Build history of the part. All positions in model axes, mm. Round coordinates to 2 decimals unless told otherwise and drop trailing zeros. Loops run counter-clockwise (first coordinate to the right, second up) from the corner with the lowest first, then second, coordinate; pieces in that order, holes last. Notation, with made-up numbers: (61, 18.5) - (82, 18.5) arc R17 ccw to (82, 47.5) - close; hole circle Ø3 at (29, 24.5). An arc over 180 degrees is marked (long way). One line per question, with ' | ' between items. Start each with the question number.
from build123d import *

# Parameters (mm, degrees)
SKETCH_1_R          = 15
EXTRUDE_1_DEPTH     = 3
M3X0_5_1_D          = 2.5
SKETCH_6_R          = 3
CUT_EXTRUDE_2_DEPTH = 22.424285286


with BuildPart() as part:
    # ｽｹｯﾁ1 → ﾎﾞｽ - 押し出し1 (new body)
    with BuildSketch(Plane(origin=(0, 0, 0), x_dir=(0, 0, -1), z_dir=(1, 0, 0))):
        Circle(SKETCH_1_R)
    extrude(amount=EXTRUDE_1_DEPTH)

    # M3x0.5 ねじ穴1 (through all)
    with Locations(Plane(origin=(3, 0, 0), x_dir=(0, 0, -1), z_dir=(1, 0, 0))):
        with Locations((-7.071067812, 7.071067812), (7.071067812, -7.071067812), (7.071067812, 7.071067812), (-7.071067812, -7.071067812)):
            Hole(M3X0_5_1_D / 2)

    # ｽｹｯﾁ6 → ｶｯﾄ - 押し出し2 (cut, through all)
    with BuildSketch(Plane(origin=(3, 0, 0), x_dir=(0, 0, -1), z_dir=(1, 0, 0))):
        Circle(SKETCH_6_R)
    extrude(amount=-CUT_EXTRUDE_2_DEPTH, mode=Mode.SUBTRACT)


solid = part.part
1) Saw through at C-C on x = 2. Write the cut outline in (y, z), and give its area (3 significant figures).
2) Two-plate mould, pull along Y, no slides. Class faces 1 (the flat face through (0, 4, 0)), 2 (the cylindrical face through (1.479, 6.31, -8.063)), 3 (the cylindrical face through (1.479, 0.66, 14.985)): +Y half, -Y half, draft (parallel to the pull), parting line (faces both ways), or undercut.
3) Saw through at D-D on z = -4.75. Write the cut outline in (x, y).
4) Saw through at A-A on z = 0. Write the cut outline in (x, y), and give its area (3 significant figures).
5) Wall check: line 1 (Z direction, x = 1.5, y = -7.75); line 2 (Y direction, x = 2.1, z = 0); line 3 (Z direction, x = 0.35, y = 8). Give the ranges that are in metal, low to high. Write a range as [from, to].
6) Drop flat-ended pins along their axis: pin 1 (5 mm diameter, centred on y = 0, z = 0, fed in from -X); pin 2 (1.5 mm diameter, centred on x = 1, y = -10.5, fed in from +Z). Give the stop position or say it passes through.
Answer key:
1) outline: circle Ø30 at (0, 0); hole circle Ø2.5 at (-7.07, -7.07); hole circle Ø2.5 at (-7.07, 7.07); hole circle Ø6 at (0, 0); hole circle Ø2.5 at (7.07, -7.07); hole circle Ø2.5 at (7.07, 7.07) | area: 659 mm²
2) face 1: draft | face 2: undercut | face 3: parting line
3) outline: (0, -14.23) - (3, -14.23) - (3, 14.23) - (0, 14.23) - close
4) outline: (0, -15) - (3, -15) - (3, -3) - (0, -3) - close; (0, 3) - (3, 3) - (3, 15) - (0, 15) - close | area: 72.0 mm²
5) line 1: [-12.84, -8.12], [-6.02, 6.02], [8.12, 12.84] | line 2: [-15, -3], [3, 15] | line 3: [-12.69, -7.91], [-6.23, 6.23], [7.91, 12.69]
6) pin 1: through | pin 2: z = 11.4
